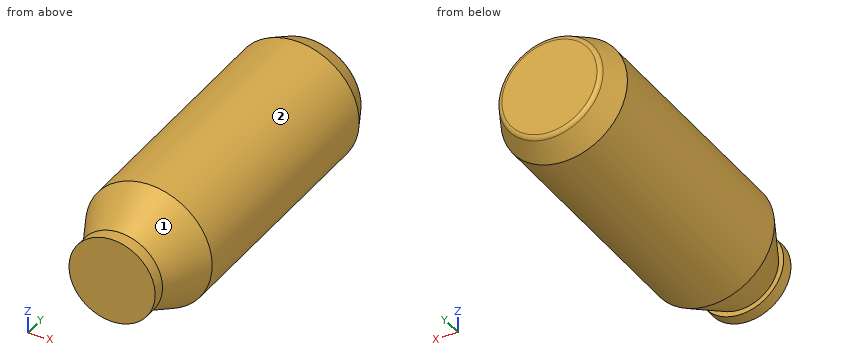
from build123d import *

# Parameters (mm, degrees)
SKETCH_3_R      = 25
EXTRUDE_2_DEPTH = 100
SKETCH_6_R      = 17
EXTRUDE_3_DEPTH = 5
FILLET_1_R      = 2


with BuildPart() as part:
    # 草图2 → 旋转1 (revolve)
    with BuildSketch(Plane(origin=(0, 0, 0), x_dir=(0, 0, -1), z_dir=(1, 0, 0))):
        Polygon((0, 0), (25, 0), (20, 10), (0, 10), align=None)
    revolve(axis=Axis((0, 0, 0), (0, 1, 0)))

    # 草图3 → 凸台-拉伸2 (add)
    with BuildSketch(Plane(origin=(0, 0, 0), x_dir=(-1, 0, 0), z_dir=(0, -1, 0))):
        Circle(SKETCH_3_R)
    extrude(amount=EXTRUDE_2_DEPTH)

    # 草图5 → 旋转2 (revolve)
    with BuildSketch(Plane(origin=(0, 0, 0), x_dir=(0, 0, -1), z_dir=(1, 0, 0))):
        Polygon((-25, -100), (0, -100), (0, -120), (-15, -120), align=None)
    revolve(axis=Axis((0, -100, 0), (0, -1, 0)))

    # 草图6 → 凸台-拉伸3 (add)
    with BuildSketch(Plane(origin=(0, -120, 0), x_dir=(-1, 0, 0), z_dir=(0, -1, 0))):
        Circle(SKETCH_6_R)
    extrude(amount=EXTRUDE_3_DEPTH)

    # 圆角1
    fillet_1_edges = [part.edges().sort_by_distance(p)[0] for p in [
        (0, 10, 20),
    ]]
    fillet(fillet_1_edges, radius=FILLET_1_R)


solid = part.part
Design review of the part built by this model. Coordinates are the model's own, in mm. Face numbers are marked on the shaded views. A direction names the side the tool comes from. Round coordinates to 2 decimals unless told otherwise and drop trailing zeros. Write each loop counter-clockwise with the first axis right and the second up, starting at its lowest first coordinate (ties: lowest second). Pieces come first, ordered by that corner, then holes. Notation, with made-up numbers: (47.5, -5.5) - (103.5, -5.5) arc R25 cw to (103.5, 6.5) - close; hole circle Ø7 at (-2, -17). An arc over 180 degrees is marked (long way). Return JSON: item names as keys, results as strings. Group by question number.
Item 1: Machinability: for the marked faces 1 and 2, which of the approach directions +Z, -Z, +X, -X, +Y, -Y give a long, thin tool a straight path to every point of the face, cutting with its end or side? Answer none if there is none.
Item 2: We need section A-A on x = 0. Write out the cut boundary in (y, z), and give its area (3 significant figures).
Item 3: We need section C-C on y = -59. Write out the cut boundary in (x, z), and give its area (3 significant figures).
Item 4: For probe 1 along Z at (x, y) = (16.5, -34.5); probe 2 along X at (y, z) = (-59.5, -15.5); probe 3 along Z at (x, y) = (-5.5, -90), list the stretches that pass through material, from the lowest coordinate up. Write a range as [from, to].
Item 5: Insertion check: P1, Ø5, axis at x = 7.5, y = -71.5, coming from the -Z side; P2, Ø5, axis at y = -88, z = -17, coming from the +X side; P3, Ø12, axis at x = -19, z = 18, coming from the +Y side. Each pin has a flat end and moves straight along its axis. Give the tip position at first contact, or say it passes through.
Item 6: We need section B-B on z = 0. Write out the cut boundary in (x, y).
Item 7: We need section D-D on y = -111. Write out the cut boundary in (x, z).
Model answer:
{
 "1": {"face 1": "none", "face 2": "+Y, -Y"},
 "2": {"outline": "(-125, -17) - (-120, -17) - (-120, -15) - (-100, -25) - (0, -25) - (8.89, -20.55) arc R2 ccw to (10, -18.76) - (10, 18.76) arc R2 ccw to (8.89, 20.55) - (0, 25) - (-100, 25) - (-120, 15) - (-120, 17) - (-125, 17) - close", "area": "6,420 mm²"},
 "3": {"outline": "circle Ø50 at (0, 0)", "area": "1,960 mm²"},
 "4": {"probe 1": "z = [-18.78, 18.78]", "probe 2": "x = [-19.62, 19.62]", "probe 3": "z = [-24.39, 24.39]"},
 "5": {"P1": "stops at z = -24.49", "P2": "stops at x = 20.37", "P3": "stops at y = 9.42"},
 "6": {"outline": "(-25, -100) - (-15, -120) - (-17, -120) - (-17, -125) - (17, -125) - (17, -120) - (15, -120) - (25, -100) - (25, 0) - (20.55, 8.89) arc R2 ccw to (18.76, 10) - (-18.76, 10) arc R2 ccw to (-20.55, 8.89) - (-25, 0) - close"},
 "7": {"outline": "circle Ø39 at (0, 0)"}
}
